```python
from build123d import *

# Parameters (mm, degrees)
BOSS_EXTRUDE1_DEPTH       = 77
FILLET1_R                 = 1
SKETCH2_W                 = 3
SKETCH2_H                 = 5
CUT_EXTRUDE1_DEPTH        = 10
LPATTERN1_COUNT           = 2
LPATTERN1_PITCH           = 3.5
LPATTERN2_COUNT           = 2
LPATTERN2_PITCH           = 60
LPATTERN2_COPY_1_SKETCH_W = 3
LPATTERN2_COPY_1_SKETCH_H = 5
LPATTERN2_COPY_1_DEPTH    = 10
LPATTERN4_COUNT           = 2
LPATTERN4_PITCH           = 53
LPATTERN4_COPY_1_SKETCH_W = 3
LPATTERN4_COPY_1_SKETCH_H = 5
LPATTERN4_COPY_1_DEPTH    = 10


with BuildPart() as part:
    # Sketch1 → Boss-Extrude1 (new body)
    with BuildSketch(Plane.XY):
        Polygon((-46.65, 0), (46.65, 0), (45.15, 27.4), (34.65, 27.4), (33.7, 46.8), (22.75, 46.8), (22.4, 55.5), (-22.4, 55.5), (-22.75, 46.8), (-33.7, 46.8), (-34.65, 27.4), (-45.15, 27.4), align=None)
    extrude(amount=BOSS_EXTRUDE1_DEPTH)

    # Fillet1
    fillet1_edges = [part.edges().sort_by_distance(p)[0] for p in [
        (-45.15, 27.4, 38.5),
        (-33.7, 46.8, 38.5),
        (-22.4, 55.5, 38.5),
        (22.4, 55.5, 38.5),
        (33.7, 46.8, 38.5),
        (45.15, 27.4, 38.5),
    ]]
    fillet(fillet1_edges, radius=FILLET1_R)

    # Sketch2 → Cut-Extrude1 (cut)
    with BuildSketch(Plane(origin=(46.65, 0, 0), x_dir=(0, 0, -1), z_dir=(1, 0, 0))):
        with Locations((-5.5, 11.5)):
            Rectangle(SKETCH2_W, SKETCH2_H)
    cut_extrude1 = extrude(amount=-CUT_EXTRUDE1_DEPTH, mode=Mode.SUBTRACT)

    # LPattern1: Cut-Extrude1 ×2
    with Locations(*[(0, 0, i * LPATTERN1_PITCH) for i in range(1, LPATTERN1_COUNT)]):
        add(cut_extrude1, mode=Mode.SUBTRACT)

    # LPattern2: Cut-Extrude1 ×2
    with Locations(*[(0, 0, i * LPATTERN2_PITCH) for i in range(1, LPATTERN2_COUNT)]):
        add(cut_extrude1, mode=Mode.SUBTRACT)

    # LPattern2 copy 1 sketch → LPattern2 copy 1 (cut)
    with BuildSketch(Plane(origin=(46.65, 0, 63.5), x_dir=(0, 0, -1), z_dir=(1, 0, 0))):
        with Locations((-5.5, 11.5)):
            Rectangle(LPATTERN2_COPY_1_SKETCH_W, LPATTERN2_COPY_1_SKETCH_H)
    extrude(amount=-LPATTERN2_COPY_1_DEPTH, mode=Mode.SUBTRACT)

    # LPattern4: Cut-Extrude1 ×2
    with Locations(*[(0, 0, i * LPATTERN4_PITCH) for i in range(1, LPATTERN4_COUNT)]):
        add(cut_extrude1, mode=Mode.SUBTRACT)

    # LPattern4 copy 1 sketch → LPattern4 copy 1 (cut)
    with BuildSketch(Plane(origin=(46.65, 0, 56.5), x_dir=(0, 0, -1), z_dir=(1, 0, 0))):
        with Locations((-5.5, 11.5)):
            Rectangle(LPATTERN4_COPY_1_SKETCH_W, LPATTERN4_COPY_1_SKETCH_H)
    extrude(amount=-LPATTERN4_COPY_1_DEPTH, mode=Mode.SUBTRACT)


solid = part.part
```
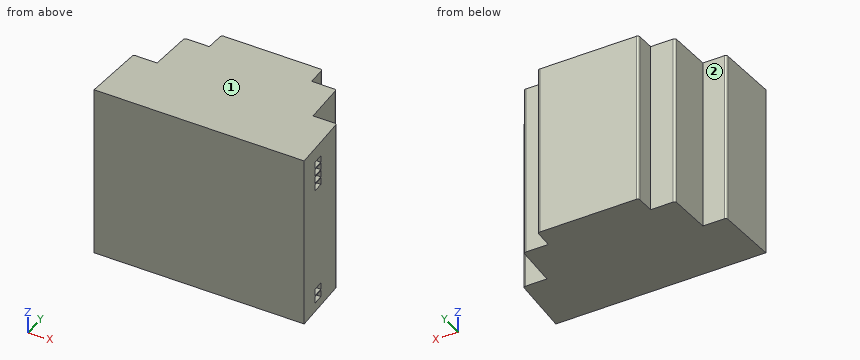
Here's how the part is built. I have some questions about the finished solid (model axes, mm). Face numbers are marked on the shaded views. A direction names the side the tool comes from. Round coordinates to 2 decimals unless told otherwise and drop trailing zeros. Write each loop counter-clockwise with the first axis right and the second up, starting at its lowest first coordinate (ties: lowest second). Pieces come first, ordered by that corner, then holes.
Q1. Please list where these lines run through material, in increasing order: probe 1 along Y at (x, z) = (41.5, 23); probe 2 along X at (y, z) = (12, 22); probe 3 along X at (y, z) = (28, 8.5).
Q2. Which directions (+Z, -Z, +X, -X, +Y, -Y) give clear straight access to the entire face, cutting with the end or side of a thin tool? Please do the marked faces 1 and 2.
Q3. If we section it at C-C on y = 40: Write out the boundary of the cut face in (x, z), plus the area to 3 significant figures.
Q4. If we section it at B-B on x = 28: Write out the boundary of the cut face in (y, z), plus the area to 3 significant figures.
Q5. If we section it at A-A on z = 54.5: Write out the boundary of the cut face in (x, y).
Q6. Will these pins go through, and if not, where does the flat tip stop? P1, Ø2.5, axis at x = 42, z = 9, coming from the +Y side; P2, Ø2.5, axis at y = 12, z = 59, coming from the +X side; P3, Ø0.9, axis at y = 12.5, z = 9.5, coming from the +X side.
Answer below:
1. probe 1: y = 0 to 27.4
1. probe 2: x = -45.99 to 45.99
1. probe 3: x = -34.62 to 34.62
2. face 1: +Z, +X, -X, +Y, -Y
2. face 2: +Z, -Z, -X, +Y
3. outline: (-34.03, 0) - (34.03, 0) - (34.03, 77) - (-34.03, 77) - close
3. area: 5,240 mm2
4. outline: (0, 0) - (46.8, 0) - (46.8, 77) - (0, 77) - close
4. area: 3,600 mm2
5. outline: (-46.65, 0) - (46.65, 0) - (45.2, 26.45) arc R1 ccw to (44.2, 27.4) - (34.65, 27.4) - (33.75, 45.85) arc R1 ccw to (32.75, 46.8) - (22.75, 46.8) - (22.44, 54.54) arc R1 ccw to (21.44, 55.5) - (-21.44, 55.5) arc R1 ccw to (-22.44, 54.54) - (-22.75, 46.8) - (-32.75, 46.8) arc R1 ccw to (-33.75, 45.85) - (-34.65, 27.4) - (-44.2, 27.4) arc R1 ccw to (-45.2, 26.45) - close
6. P1: stops at y = 27.4
6. P2: stops at x = 46.03
6. P3: stops at x = 36.65
